Read the model definition and answer for the solid it produces. Units are mm, in the model's axes. A direction names the side the tool comes from. Give positions to 0.01 mm unless a question says otherwise; leave off trailing zeros. Loops run counter-clockwise (first coordinate to the right, second up) from the corner with the lowest first, then second, coordinate; pieces in that order, holes last. Notation, with made-up numbers: (21.25, 57) -> (49.25, 57) arc R31 ccw to (49.25, 94) -> close; hole circle Ø5 at (59.25, 59.5). An arc over 180 degrees is marked (long way). Answer as CSV lines item,"result". Start each with the question number.
```python
from build123d import *

# Parameters (mm, degrees)
BOSS_EXTRU_1_DEPTH                                 = 20
ESQUISSE19_W                                       = 4.8
ESQUISSE19_H                                       = 21.581272728
ENL_V_MAT_EXTRU_1_DEPTH                            = 6.25
CHAMBRAGE_POUR_VIS_T_TE_RONDE_BOMB_E_M_D           = 3.4
CHAMBRAGE_POUR_VIS_T_TE_RONDE_BOMB_E_M_CBORE_D     = 7
CHAMBRAGE_POUR_VIS_T_TE_RONDE_BOMB_E_M_CBORE_DEPTH = 2.4
D_GAGEMENT_M41_D                                   = 4.5


with BuildPart() as part:
    # Base → Boss.-Extru.1 (new, symmetric)
    with BuildSketch(Plane(origin=(0, 0, 0), x_dir=(1, 0, 0), z_dir=(0, 1, 0))):
        Polygon((-3, 10.061730862), (-2.4, 10.061730862), (-2.4, 3.811730862), (2.4, 3.811730862), (2.4, 10.061730862), (3, 10.061730862), (22.5, 10.061730862), (22.5, 15.361730862), (-22.5, 15.361730862), (-22.5, 10.061730862), align=None)
    extrude(amount=BOSS_EXTRU_1_DEPTH, both=True)

    # Esquisse19 → Enlèv. mat.-Extru.1 (cut)
    with BuildSketch(Plane.XY.offset(-3.811730862)):
        with Locations((0, -3.896618687)):
            Rectangle(ESQUISSE19_W, ESQUISSE19_H)
    extrude(amount=-ENL_V_MAT_EXTRU_1_DEPTH, mode=Mode.SUBTRACT)

    # Chambrage pour vis à tête ronde bombée M31 (through all)
    with Locations(Plane.XY.offset(-10.061730862)):
        with Locations((-14, 14.142273416), (14, 14.142273416), (0, -10.857726584)):
            CounterBoreHole(CHAMBRAGE_POUR_VIS_T_TE_RONDE_BOMB_E_M_D / 2, CHAMBRAGE_POUR_VIS_T_TE_RONDE_BOMB_E_M_CBORE_D / 2, CHAMBRAGE_POUR_VIS_T_TE_RONDE_BOMB_E_M_CBORE_DEPTH)

    # Dégagement M41 (through all)
    with Locations(Plane(origin=(0, 0, -15.361730862), x_dir=(-1, 0, 0), z_dir=(0, 0, -1))):
        with Locations((0, 0)):
            Hole(D_GAGEMENT_M41_D / 2)


solid = part.part
```
(1) Find section A-A on x = -14. Write down the section's boundary in (y, z).
(2) Each of these flat-tipped pins is pushed along its axis until it touches: P1, Ø1.6, axis at y = -18, z = -5.5, coming from the -X side; P2, Ø3, axis at x = -8, y = 8, coming from the +Z side; P3, Ø3.5, axis at x = 15, y = 15.5, coming from the +Z side; P4, Ø2, axis at x = -14, y = 14.14, coming from the +Z side. Where does it stop, or does it pass through?
(3) Find section D-D on z = -5.25. Write down the section's boundary in (x, y), then the cut area to 3 significant figures.
(4) The mould has two halves that part along X. Classify faces 5 (the face through (0, -14.687, -7)), 6 (the face through (-10.66, 15.19, -11.24)), 7 (the face through (2.4, -17, -7)), 8 (the face through (-22.5, 0, -13)): pulls with the +X half, pulls with the -X half, needs draft (parallel to the pull), parting line crosses it, or undercut.
(5) Find section C-C on x = 0. Write down the section's boundary in (y, z).
(6) A tool of negligible diameter and unlimited length cuts with its end or side. For faces 1 (the face through (2, -10, -12.462)), 2 (the face through (-2.4, -17, -7)), 3 (the face through (2.4, 14, -7)), 4 (the face through (0, 6.894, -7)), from which of +Z, -Z, +X, -X, +Y, -Y can it reach the whole face along a straight path? Write none if from no direction.
(7) Find section B-B on y = 0. Write down the section's boundary in (x, z).
(8) Find the intervals of material crossed by line 1 along Y through (x, z) = (2, -6.5); line 2 along Y through (x, z) = (14, -11.15); line 3 along Y through (x, z) = (-1.5, -12.25), in increasing order. Write a range as from..to.
Answer block:
1,outline,"(-20, -15.36) -> (12.44, -15.36) -> (12.44, -12.46) -> (10.64, -12.46) -> (10.64, -10.06) -> (-20, -10.06) -> close; (15.84, -15.36) -> (20, -15.36) -> (20, -10.06) -> (17.64, -10.06) -> (17.64, -12.46) -> (15.84, -12.46) -> close"
2,P1,"stops at x = -2.4"
2,P2,"stops at z = -10.06"
2,P3,"stops at z = -12.46"
2,P4,"passes through"
3,outline,"(-2.4, -20) -> (2.4, -20) -> (2.4, -14.69) -> (-2.4, -14.69) -> close; (-2.4, 6.89) -> (2.4, 6.89) -> (2.4, 20) -> (-2.4, 20) -> close"
3,area,"88.4 mm2"
4,face 5,"needs draft"
4,face 6,"undercut"
4,face 7,"pulls with the +X half"
4,face 8,"pulls with the -X half"
5,outline,"(-20, -15.36) -> (-12.56, -15.36) -> (-12.56, -12.46) -> (-14.36, -12.46) -> (-14.36, -10.06) -> (-14.69, -10.06) -> (-14.69, -3.81) -> (-20, -3.81) -> close; (-9.16, -15.36) -> (-2.25, -15.36) -> (-2.25, -10.06) -> (-7.36, -10.06) -> (-7.36, -12.46) -> (-9.16, -12.46) -> close; (2.25, -15.36) -> (20, -15.36) -> (20, -3.81) -> (6.89, -3.81) -> (6.89, -10.06) -> (2.25, -10.06) -> close"
6,face 1,"+Z"
6,face 2,"+Z, -X, +Y, -Y"
6,face 3,"+Z, +X, +Y, -Y"
6,face 4,"+Z, +X, -X"
7,outline,"(-22.5, -15.36) -> (-2.25, -15.36) -> (-2.25, -10.06) -> (-22.5, -10.06) -> close; (2.25, -15.36) -> (22.5, -15.36) -> (22.5, -10.06) -> (2.25, -10.06) -> close"
8,line 1,"y = -20..-14.69, 6.89..20"
8,line 2,"y = -20..10.64, 17.64..20"
8,line 3,"y = -20..-14.02, -7.7..-1.68, 1.68..20"
